The model under review builds one solid part; all positions refer to its coordinate system, in mm. Give positions to 0.01 mm unless a question says otherwise; leave off trailing zeros. Order: outer loops, then holes, each group sorted by start corner. A loop starts at its lowest first (then second) coordinate and runs counter-clockwise, first axis right, second up.
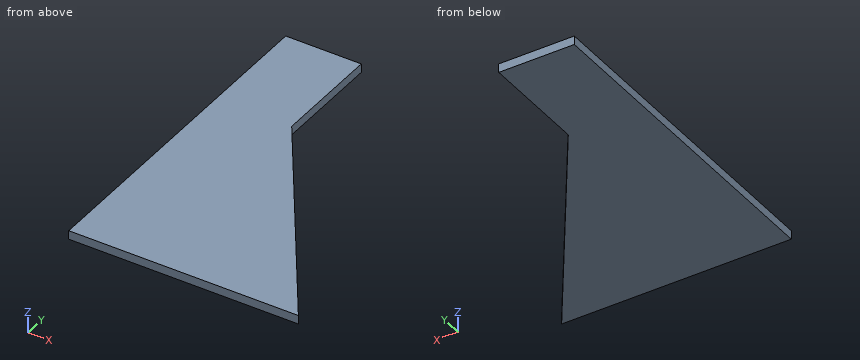
```python
from build123d import *

# Parameters (mm, degrees)
BOSS_EXTRUDE1_DEPTH = 3


with BuildPart() as part:
    # Sketch1 → Boss-Extrude1 (new body)
    with BuildSketch(Plane.XY.offset(-231.833966153)):
        Polygon((0, 0), (0, -116.353177225), (79.018807169, -116.353177225), (26, -37.313053542), (26, 0), align=None)
    extrude(amount=-BOSS_EXTRUDE1_DEPTH)


solid = part.part
```
Item 1: Clearance check with a flat-ended pin moving along its axis: pin 1 Ø1 at (y, z) = (-53.5, -232) entering from +X. State where the tip first meets the part, or that it passes through.
Values found:
pin 1: stops at x = 37.19
Item 2: Take a section at A-A (z = -232.4). Give the boundary of the cut face in (x, y), and give its area (3 significant figures).
Values found:
outline: (0, -116.35) - (79.02, -116.35) - (26, -37.31) - (26, 0) - (0, 0) - close
area: 5,120 mm2
Item 3: Take a section at C-C (x = 66.5). Give the boundary of the cut face in (y, z), and give its area (3 significant figures).
Values found:
outline: (-116.35, -234.83) - (-97.69, -234.83) - (-97.69, -231.83) - (-116.35, -231.83) - close
area: 56.0 mm2
Item 4: For line 1 (X direction, y = -32.5, z = -232.3); line 2 (X direction, y = -86, z = -233.15); line 3 (Y direction, x = 53.5, z = -234.2), list the stretches that pass through material, from the lowest coordinate up.
Values found:
line 1: x = 0 to 26
line 2: x = 0 to 58.66
line 3: y = -116.35 to -78.31
Item 5: Take a section at B-B (y = -35.5). Give the boundary of the cut face in (x, z), and give its area (3 significant figures).
Values found:
outline: (0, -234.83) - (26, -234.83) - (26, -231.83) - (0, -231.83) - close
area: 78.0 mm2
